Design review of the part built by this model. Coordinates are the model's own, in mm. A direction names the side the tool comes from. Give positions to 0.01 mm unless a question says otherwise; leave off trailing zeros. Loops run counter-clockwise (first coordinate to the right, second up) from the corner with the lowest first, then second, coordinate; pieces in that order, holes last. Notation, with made-up numbers: (47.5, 22) - (81.5, 22) arc R14 cw to (81.5, 49) - close; hole circle Ø10 at (29.5, 20). An arc over 180 degrees is marked (long way). Put each result on its own line as item: value. Start each with the question number.
```python
from build123d import *

# Parameters (mm, degrees)
F0_W     = 254
F0_H     = 152.4
F0_R     = 2.2479
F0_R_2   = 1.7272
F0_W_2   = 76.2
F0_H_2   = 76.2
F0_R_3   = 3.175
F1_DEPTH = 6.35


with BuildPart() as f1:
    # F0 (on Top) → F1 (new body)
    with BuildSketch(Plane.XY):
        Rectangle(F0_W, F0_H)
        with Locations((-114.3, -63.5)):
            Circle(F0_R, mode=Mode.SUBTRACT)
        with Locations((-95.25, -63.5)):
            Circle(F0_R_2, mode=Mode.SUBTRACT)
        with Locations((-6.35, -63.5)):
            Circle(F0_R_2, mode=Mode.SUBTRACT)
        with Locations((-50.8, -19.05)):
            Rectangle(F0_W_2, F0_H_2, mode=Mode.SUBTRACT)
        with Locations((114.3, -63.5)):
            Circle(F0_R, mode=Mode.SUBTRACT)
        with Locations((25.4, -6.35)):
            Circle(F0_R_3, mode=Mode.SUBTRACT)
        with Locations((81.534, -25.4)):
            Circle(F0_R_2, mode=Mode.SUBTRACT)
        with Locations((96.774, -25.4)):
            Circle(F0_R_2, mode=Mode.SUBTRACT)
        with Locations((-95.25, 25.4)):
            Circle(F0_R_2, mode=Mode.SUBTRACT)
        with Locations((-6.35, 25.4)):
            Circle(F0_R_2, mode=Mode.SUBTRACT)
        with Locations((-114.3, 63.5)):
            Circle(F0_R, mode=Mode.SUBTRACT)
        with Locations((114.3, 63.5)):
            Circle(F0_R, mode=Mode.SUBTRACT)
    extrude(amount=F1_DEPTH)


solid = f1.part
```
Item 1: Consider section B-B (x = 25.4). State the section outline as (y, z) points (3 decimals), plus the area to 3 significant figures.
Item 2: Machinability: for faces 4 (the flat face through (-2, 1, 6.35)), 5 (the flat face through (-51, 19.05, 3)), which of the approach directions +Z, -Z, +X, -X, +Y, -Y give a long, thin tool a straight path to every point of the face, cutting with its end or side? Answer none if there is none.
Item 3: Consider section A-A (y = -6.35). State the section outline as (x, z) points (3 decimals), plus the area to 3 significant figures.
Item 4: Consider section C-C (z = 5.25). Count the separate pieces of the cut face and the enclosed holes in it, plus the area to 3 significant figures.
Item 5: Mouldability with a two-part tool opening along Y and no side actions: class faces 1 (the flat face through (-2, 1, 0)), 2 (the flat face through (-2, -76.2, 3)), 3 (the cylindrical face through (116.376, -64.361, 3.131)) as pulls with the +Y half, pulls with the -Y half, needs draft (parallel to the pull), parting line crosses it, or undercut.
Item 6: For L1, parallel to Y at x = -6.35, z = 2.75; L2, parallel to Y at x = -114.3, z = 4.25; L3, parallel to X at y = -6.5, z = 1.5, list the stretches that pass through material, from the lowest coordinate up. Write a range as from..to.
Item 7: Consider section D-D (x = -25.5). State the section outline as (y, z) points.
Geometry says:
1. outline: (-76.2, 0) - (-9.525, 0) - (-9.525, 6.35) - (-76.2, 6.35) - close; (-3.175, 0) - (76.2, 0) - (76.2, 6.35) - (-3.175, 6.35) - close
1. area: 927 mm2
2. face 4: +Z, +X, -X, +Y, -Y
2. face 5: +Z, -Z
3. outline: (-127, 0) - (-88.9, 0) - (-88.9, 6.35) - (-127, 6.35) - close; (-12.7, 0) - (22.225, 0) - (22.225, 6.35) - (-12.7, 6.35) - close; (28.575, 0) - (127, 0) - (127, 6.35) - (28.575, 6.35) - close
3. area: 1,090 mm2
4. separate pieces: 1
4. enclosed holes: 12
4. area: 32,800 mm2
5. face 1: needs draft
5. face 2: pulls with the -Y half
5. face 3: undercut
6. L1: y = -76.2..-65.23, -61.77..23.67, 27.13..76.2
6. L2: y = -76.2..-65.75, -61.25..61.25, 65.75..76.2
6. L3: x = -127..-88.9, -12.7..22.23, 28.57..127
7. outline: (-76.2, 0) - (-57.15, 0) - (-57.15, 6.35) - (-76.2, 6.35) - close; (19.05, 0) - (76.2, 0) - (76.2, 6.35) - (19.05, 6.35) - close
